from build123d import *

# Parameters (mm, degrees)
BOSS_EXTRUDE1_DEPTH             = 32
SKETCH3_OUTSIDE_W               = 82.906
SKETCH3_OUTSIDE_H               = 63.906
CUT_EXTRUDE1_DEPTH              = 22
SKETCH6_R                       = 6
CUT_EXTRUDE2_DEPTH              = 24
CUT_EXTRUDE3_REACH              = 65.82
CUT_EXTRUDE3_END_RADIUS         = 6
SKETCH7_R                       = 3
SKETCH8_R                       = 5
CUT_EXTRUDE4_DEPTH              = 4
M6X1_0_TAPPED_HOLE2_D           = 5
M6X1_0_TAPPED_HOLE2_DEPTH       = 16
M6X1_0_TAPPED_HOLE2_CSINK_D     = 6.05
M6X1_0_TAPPED_HOLE2_CSINK_ANGLE = 100
M6X1_0_TAPPED_HOLE2_TIP         = 1.502151548
FILLET1_R                       = 3


with BuildPart() as part:
    # Sketch1 → Boss-Extrude1 (new body)
    with BuildSketch(Plane(origin=(0, 0, 0), x_dir=(0, 0, -1), z_dir=(1, 0, 0))):
        Polygon((8, -18), (32, -18), (32, 18), (-32, 18), (-32, -18), (-8, -18), (-8, -27), (8, -27), align=None)
    extrude(amount=-BOSS_EXTRUDE1_DEPTH)

    # Sketch3 outside → Cut-Extrude1 (cut)
    with BuildSketch(Plane(origin=(0, 0, 0), x_dir=(0, 0, -1), z_dir=(1, 0, 0))):
        with Locations((0, -4.5)):
            Rectangle(SKETCH3_OUTSIDE_W, SKETCH3_OUTSIDE_H)
        with BuildLine():
            Line((-27.5, -8), (-12.8, 11.6))
            ThreePointArc((-12.8, 11.6), (0, 18), (12.8, 11.6))
            Line((12.8, 11.6), (27.5, -8))
            Line((27.5, -8), (32, -8))
            Line((32, -8), (32, -18))
            Line((32, -18), (8, -18))
            Line((8, -18), (8, -27))
            Line((8, -27), (-8, -27))
            Line((-8, -27), (-8, -18))
            Line((-8, -18), (-32, -18))
            Line((-32, -18), (-32, -8))
            Line((-32, -8), (-27.5, -8))
        make_face(mode=Mode.SUBTRACT)
    extrude(amount=-CUT_EXTRUDE1_DEPTH, mode=Mode.SUBTRACT)

    # Sketch6 → Cut-Extrude2 (cut)
    with BuildSketch(Plane(origin=(0, 0, 0), x_dir=(0, 0, -1), z_dir=(1, 0, 0))):
        with Locations((0, 2)):
            Circle(SKETCH6_R)
    extrude(amount=-CUT_EXTRUDE2_DEPTH, mode=Mode.SUBTRACT)

    # Cut-Extrude3: up to this cylinder (the profile starts outside it)
    cut_extrude3_end = Plane(origin=(-12, 2, 0), z_dir=(1, 0, 0)) * Cylinder(CUT_EXTRUDE3_END_RADIUS, 144.64, mode=Mode.PRIVATE)
    # Sketch7 → Cut-Extrude3 (cut, up to the surface)
    with BuildSketch(Plane(origin=(0, 18, 0), x_dir=(1, 0, 0), z_dir=(0, 1, 0)), mode=Mode.PRIVATE) as cut_extrude3_sk1:
        with Locations(Location((-12, 0, 0), (0, 0, 270))):
            Circle(SKETCH7_R)
    cut_extrude3_tool1 = extrude(cut_extrude3_sk1.sketch, amount=-CUT_EXTRUDE3_REACH, mode=Mode.PRIVATE) - cut_extrude3_end
    add(cut_extrude3_tool1.solids().sort_by_distance((-12, 18, 0))[0], mode=Mode.SUBTRACT)

    # Sketch8 → Cut-Extrude4 (cut)
    with BuildSketch(Plane(origin=(0, 18, 0), x_dir=(1, 0, 0), z_dir=(0, 1, 0))):
        with Locations(Location((-12, 0, 0), (0, 0, 270))):
            Circle(SKETCH8_R)
    extrude(amount=-CUT_EXTRUDE4_DEPTH, mode=Mode.SUBTRACT)

    # M6x1.0 Tapped Hole2
    with Locations(Plane(origin=(0, -27, 0), x_dir=(-1, 0, 0), z_dir=(0, -1, 0))):
        with Locations((8, 0), (24, 0)):
            CounterSinkHole(M6X1_0_TAPPED_HOLE2_D / 2, M6X1_0_TAPPED_HOLE2_CSINK_D / 2, depth=M6X1_0_TAPPED_HOLE2_DEPTH, counter_sink_angle=M6X1_0_TAPPED_HOLE2_CSINK_ANGLE)
            with Locations((0, 0, -(M6X1_0_TAPPED_HOLE2_DEPTH + M6X1_0_TAPPED_HOLE2_TIP / 2))):  # 118° drill point
                Cone(0, M6X1_0_TAPPED_HOLE2_D / 2, M6X1_0_TAPPED_HOLE2_TIP, mode=Mode.SUBTRACT)

    # Fillet1
    fillet1_edges = [part.edges().sort_by_distance(p)[0] for p in [
        (-11, -8, 27.5),
        (-11, -8, -27.5),
    ]]
    fillet(fillet1_edges, radius=FILLET1_R)


solid = part.part
Design review of the part built by this model. Coordinates are the model's own, in mm. A direction names the side the tool comes from. Coordinates: 2 decimals unless noted, no trailing zeros. Loops run counter-clockwise (first coordinate to the right, second up) from the corner with the lowest first, then second, coordinate; pieces in that order, holes last.
Item 1: Add section C-C (y = 2). Write out the cut boundary in (x, z).
Completed:
outline: (-32, -32) - (-22, -32) - (-22, -20) - (0, -20) - (0, -6) - (-24, -6) - (-24, 6) - (0, 6) - (0, 20) - (-22, 20) - (-22, 32) - (-32, 32) - close
Item 2: Wall thickness on L1, parallel to X at y = 11, z = 0; L2, parallel to Z at x = -16.5, y = -21; L3, parallel to Z at x = -9.5, y = -1.5 (3 decimals): over which ranges is each line inside the solid? List them lowest first.
Completed:
L1: x = -32 to -15, -9 to 0
L2: z = -8 to 8
L3: z = -22.625 to -4.873, 4.873 to 22.625
Item 3: Draft analysis for pull direction X (two halves, no side actions). For faces 1 (the flat face through (0, -4.2, 0.4)), 2 (the cylindrical face through (-15, 16, -4)), 3 (the flat face through (-10.85, 2.53, -19.6)), state which applies: pulls with the +X half, pulls with the -X half, needs draft (parallel to the pull), parting line crosses it, or undercut.
Completed:
face 1: pulls with the +X half
face 2: undercut
face 3: needs draft
Item 4: Add section B-B (y = -20.5). Write out the cut boundary in (x, z), and give its area (3 significant figures).
Completed:
outline: (-32, -8) - (0, -8) - (0, 8) - (-32, 8) - close; hole circle Ø5 at (-24, 0); hole circle Ø5 at (-8, 0)
area: 473 mm2
Item 5: Clearance check with flat-ended pins moving along their axes: pin 1 (3 mm diameter, centred on x = -12.5, z = 0.5, fed in from +Y); pin 2 (2.5 mm diameter, centred on x = -10, z = -30, fed in from +Y); pin 3 (9.5 mm diameter, centred on y = 2.5, z = 1, fed in from +X). State where each tip first meets the part, or that it passes through.
Completed:
pin 1: stops at y = -3.66
pin 2: stops at y = -7.99
pin 3: stops at x = -24
Item 6: Add section D-D (y = 9.5). Write out the cut boundary in (x, z) (3 decimals).
Completed:
outline: (-32, -32) - (-22, -32) - (-22, -14.375) - (0, -14.375) - (0, 14.375) - (-22, 14.375) - (-22, 32) - (-32, 32) - close; hole circle Ø6 at (-12, 0)
Item 7: Add section A-A (x = -19). Write out the cut boundary in (y, z).
Completed:
outline: (-27, -8) - (-18, -8) - (-18, -32) - (-8, -32) - (-8, -29) arc R3 cw to (-6.8, -26.6) - (11.6, -12.8) arc R16 ccw to (11.6, 12.8) - (-6.8, 26.6) arc R3 cw to (-8, 29) - (-8, 32) - (-18, 32) - (-18, 8) - (-27, 8) - close; hole circle Ø12 at (2, 0)
Item 8: For faces 4 (the cylindrical face through (-12, 11, -3)), 5 (the flat face through (-16, -18, -20)), 6 (the flat face through (-16, -22, 8)), 7 (the cylindrical face through (-11.154, -7.692, 27.676)), list the 3-axis set-ups (+Z, -Z, +X, -X, +Y, -Y) from which the entire face can be reached by the end or side of a thin tool; tool diameter is ignored.
Completed:
face 4: +Y
face 5: -Z, +X, -X, -Y
face 6: +Z, +X, -X, -Y
face 7: +Z, +X, +Y
